Input: part model. Units: mm. Frame: model coordinates. A direction names the side the tool comes from. Round coordinates to 2 decimals unless told otherwise and drop trailing zeros. Order: outer loops, then holes, each group sorted by start corner. A loop starts at its lowest first (then second) coordinate and runs counter-clockwise, first axis right, second up. Notation, with made-up numbers: (48.25, 22.25) -> (75.25, 22.25) arc R17 ccw to (75.25, 30.25) -> close; hole circle Ø7 at (33, 60). An arc over 180 degrees is marked (long way). Answer as CSV lines item,"result". Start each with the question number.
1) Mould query, pull axis X, two halves, no side actions, for faces 1 (the face through (1.2, 0, 1.2)), 2 (the face through (2.726, 1.728, -0.858)), 3 (the face through (0, 1, 1.389)). Classes: +X half, -X half, draft (parallel to the pull), parting line (faces both ways), or undercut.
2) Section query D-D, the plane z = -2.1. Output: boundary loops of the cut face in (x, y), and give its area (3 significant figures).
3) Section query C-C, the plane y = 16.5. Output: boundary loops of the cut face in (x, z).
4) Access query for faces 4 (the face through (0, 1.956, 0)), 5 (the face through (-0.372, 12.897, 1.674)), 6 (the face through (0, 22.555, 0)). Directions: +Z, -Z, +X, -X, +Y, -Y. A direction counts if a zero-diameter tool reaches every point of the face in a straight line with its end or side. Return the directions, or none.
5) Line query: L1, parallel to Z at x = -0.4, y = 1.75; L2, parallel to Y at x = 0.6, z = 0.65; L3, parallel to Y at x = 0.3, z = -1.85. Output: solid intervals per line, ascending.
6) Section query B-B, the plane z = 0.75. Output: boundary loops of the cut face in (x, y).
7) Section query A-A, the plane x = 0. Output: boundary loops of the cut face in (y, z), and give its area (3 significant figures).
8) First-contact query: P1, Ø3, axis at x = 1, y = 12, coming from the -Z side; P2, Ø0.5, axis at x = 0.5, y = 1, coming from the -Z side. Flat tips, straight axial feed; report the tip coordinate or a pass-through.
```python
from build123d import *

# Parameters (mm, degrees)
SKETCH1_R           = 2.8575
BOSS_EXTRUDE1_DEPTH = 3.5052
CUT_EXTRUDE1_DEPTH  = 1.9558
SKETCH3_R           = 1.7145
BOSS_EXTRUDE2_DEPTH = 19.05


with BuildPart() as part:
    # Sketch1 → Boss-Extrude1 (new body)
    with BuildSketch(Plane(origin=(0, 0, 0), x_dir=(1, 0, 0), z_dir=(0, 1, 0))):
        Circle(SKETCH1_R)
    extrude(amount=BOSS_EXTRUDE1_DEPTH)

    # Sketch2 → Cut-Extrude1 (cut)
    with BuildSketch(Plane.XZ):
        Polygon((1.603951217, 0), (0.801975608, 1.3890625), (-0.801975608, 1.3890625), (-1.603951217, 0), (-0.801975608, -1.3890625), (0.801975608, -1.3890625), align=None)
    extrude(amount=-CUT_EXTRUDE1_DEPTH, mode=Mode.SUBTRACT)

    # Sketch3 → Boss-Extrude2 (add)
    with BuildSketch(Plane(origin=(0, 3.5052, 0), x_dir=(1, 0, 0), z_dir=(0, 1, 0))):
        Circle(SKETCH3_R)
    extrude(amount=BOSS_EXTRUDE2_DEPTH)


solid = part.part
```
Findings:
1,face 1,"draft"
1,face 2,"parting line"
1,face 3,"undercut"
2,outline,"(-1.94, 0) -> (1.94, 0) -> (1.94, 3.51) -> (-1.94, 3.51) -> close"
2,area,"13.6 mm^2"
3,outline,"circle Ø3.43 at (0, 0)"
4,face 4,"-Y"
4,face 5,"+Y"
4,face 6,"+Z, -Z, +X, -X, +Y"
5,L1,"z = -2.83 to -1.39, 1.39 to 2.83"
5,L2,"y = 1.96 to 22.56"
5,L3,"y = 0 to 3.51"
6,outline,"(-2.76, 0) -> (-1.17, 0) -> (-1.17, 1.96) -> (1.17, 1.96) -> (1.17, 0) -> (2.76, 0) -> (2.76, 3.51) -> (1.54, 3.51) -> (1.54, 22.56) -> (-1.54, 22.56) -> (-1.54, 3.51) -> (-2.76, 3.51) -> close"
7,outline,"(0, -2.86) -> (3.51, -2.86) -> (3.51, -1.71) -> (22.56, -1.71) -> (22.56, 1.71) -> (3.51, 1.71) -> (3.51, 2.86) -> (0, 2.86) -> (0, 1.39) -> (1.96, 1.39) -> (1.96, -1.39) -> (0, -1.39) -> close"
7,area,"79.9 mm^2"
8,P1,"stops at z = -1.71"
8,P2,"stops at z = -2.85"
